Read the model definition and answer for the solid it produces. Units are mm, in the model's axes. A direction names the side the tool comes from. Coordinates: 2 decimals unless noted, no trailing zeros. Write each loop counter-clockwise with the first axis right and the second up, starting at its lowest first coordinate (ties: lowest second). Pieces come first, ordered by that corner, then holes. Notation, with made-up numbers: (-30.75, -24) -> (15.25, -24) arc R23 cw to (15.25, 11) -> close; hole circle Ø4 at (17, -32.5). An arc over 180 degrees is marked (long way). One line per item, written item: value. Start each with the question number.
1. Find section A-A, the plane x = 31.5. Write down the section's boundary in (y, z).
2. For a pull along X with two mould halves and no side action, classify faces 1 (the flat face through (2, -62, 70)), 2 (the flat face through (0, -63, 35)), 3 (the flat face through (5, -120, 60.75)) as pulls with the +X half, pulls with the -X half, needs draft (parallel to the pull), parting line crosses it, or undercut.
3. Consider line 1 along Y through (x, z) = (4.75, 64.5); line 2 along X through (y, z) = (-48.5, 35); line 3 along Y through (x, z) = (30.5, 54). Determine where each line is inside the solid, lowest interval first.
4. For faces 4 (the cylindrical face through (1.5, -70.4, 31.3)), 5 (the cylindrical face through (13.65, -1.52, 34.71)), 6 (the flat face through (6, -119, 66.75)), determine the directions among +Z, -Z, +X, -X, +Y, -Y from which every point of the face is accessible in a straight line to the end or side of a thin tool.
5. Find section C-C, the plane y = -98. Write down the section's boundary in (x, z).
6. Find section B-B, the plane z = 56. Write down the section's boundary in (x, y).
7. Given P1, Ø0.6, axis at x = 9.5, y = -9, coming from the +Z side; P2, Ø1.6, axis at x = 90, y = -81, coming from the +Z side, each flat-ended and moving along its own axis, determine where each tip first touches the part or whether it passes through.
8. Find section D-D, the plane x = 75.5. Write down the section's boundary in (y, z).
Autodesk Inventor part; units mm, degrees
ref_plane "Plano de trabajo2" through (0, 0, 60.25) normal (0, 0, 1) x (1, 0, 0)
ref_plane "YZ Plane" through (0, 0, 0) normal (1, 0, 0) x (0, 1, 0)
ref_plane "XZ Plane" through (0, 0, 0) normal (0, 1, 0) x (-1, 0, 0)
sketch "Boceto3" plane through (0, 0, 0) normal (0, 0, 1) x (1, 0, 0)
  line L0 (0, 0) -> (100, 0)
  line L1 (100, 0) -> (100, -125)
  line L2 (100, -125) -> (0, -125)
  line L3 (0, -125) -> (0, 0)
  dimension "d8" = 100
  dimension "d9" = 125
extrude "Extrusión2" add sketch "Boceto3" along normal blind 70
sketch "Boceto4" plane through (0, 0, 70) normal (0, 0, 1) x (1, 0, 0)
  line L0 (0, 0) -> (50, 0)
  line L1 (100, 0) -> (0, 0)
  line L2 (0, 0) -> (0, -125)
  line L3 (0, 0) -> (0, -45)
  line L4 (6.25, -5.5) -> (93.75, -5.5)
  line L5 (93.75, -5.5) -> (93.75, -84.5)
  line L6 (93.75, -84.5) -> (6.25, -84.5)
  line L7 (6.25, -84.5) -> (6.25, -5.5)
  line L8 (6.25, -5.5) -> (93.75, -84.5) construction
  line L9 (93.75, -5.5) -> (6.25, -84.5) construction
  line L10 (6.25, -5.5) -> (9.75, -5.5)
  line L11 (6.25, -5.5) -> (6.25, -9)
  circle A0 centre (9.75, -9) radius 1
  line L12 (93.75, -5.5) -> (90.25, -5.5)
  line L13 (93.75, -5.5) -> (93.75, -9)
  circle A1 centre (90.25, -9) radius 1
  line L14 (93.75, -84.5) -> (90.25, -84.5)
  line L15 (93.75, -84.5) -> (93.75, -81)
  circle A2 centre (90.25, -81) radius 1
  line L16 (6.25, -84.5) -> (9.75, -84.5)
  line L17 (6.25, -84.5) -> (6.25, -81)
  circle A3 centre (9.75, -81) radius 1
  point P0 (50, -45)
  dimension "d12" = 45
  dimension "d13" = 87.5
  dimension "d14" = 79
  dimension "d22" = 3.5
  dimension "d23" = 3.5
  dimension "d24" = 2
  dimension "d25" = 3.5
  dimension "d26" = 3.5
  dimension "d27" = 2
  dimension "d28" = 3.5
  dimension "d29" = 3.5
  dimension "d30" = 2
  dimension "d31" = 3.5
  dimension "d32" = 3.5
  dimension "d33" = 2
sketch "Boceto5" plane through (0, 0, 70) normal (0, 0, 1) x (1, 0, 0)
  line L0 (100, 0) -> (0, 0)
  line L1 (0, 0) -> (0, -62.5)
  line L2 (0, 0) -> (0, -125)
  line L3 (0, 0) -> (3, 0)
  line L4 (0, 0) -> (0, -3)
  line L5 (100, -125) -> (100, 0)
  line L6 (100, -125) -> (100, -122)
  line L7 (0, -125) -> (100, -125)
  line L8 (100, -125) -> (97, -125)
  line L9 (97, -122) -> (3, -122)
  line L10 (3, -122) -> (3, -3)
  line L11 (3, -3) -> (97, -3)
  line L12 (97, -3) -> (97, -122)
  dimension "d15" = 62.5
  dimension "d16" = 3
  dimension "d17" = 3
  dimension "d18" = 3
  dimension "d19" = 3
extrude "Extrusión3" cut sketch "Boceto5" against normal blind 60 contours L9 L10 L11 L12
extrude "Extrusión4" cut sketch "Boceto4" against normal blind 65 contours A0 | A1 | A2 | A3
sketch "Boceto7" plane through (0, 0, 70) normal (0, 0, 1) x (1, 0, 0)
  point P0 (0, 0)
sketch "Boceto8" plane through (0, 0, 70) normal (0, 0, 1) x (1, 0, 0)
  point P0 (0, 0)
ref_plane "Plano de trabajo1" through (0, 0, 60.75) normal (0, 0, 1) x (1, 0, 0)
sketch "Boceto9" plane through (0, 0, 60.75) normal (0, 0, 1) x (1, 0, 0)
  line L0 (3, -3) -> (6.5, -3)
  line L1 (6.5, -3) -> (6.5, -6.5)
  line L2 (6.5, -6.5) -> (3, -6.5)
  line L3 (3, -6.5) -> (3, -3)
  line L4 (97.0016, -3) -> (93.5016, -3)
  line L5 (93.5016, -3) -> (93.5016, -6.5)
  line L6 (93.5016, -6.5) -> (97.0016, -6.5)
  line L7 (97.0016, -6.5) -> (97.0016, -3)
  line L8 (3, -122) -> (3, -3)
  line L9 (3, -122) -> (6.5, -122)
  line L10 (6.5, -122) -> (6.5, -118.5)
  line L11 (6.5, -118.5) -> (3, -118.5)
  line L12 (3, -118.5) -> (3, -122)
  line L13 (97, -3) -> (97, -122)
  line L14 (97, -122) -> (93.5, -122)
  line L15 (93.5, -122) -> (93.5, -118.5)
  line L16 (93.5, -118.5) -> (97, -118.5)
  line L17 (97, -118.5) -> (97, -122)
  point P0 (0, 0)
  point P1 (97, -6.5)
  dimension "d61" = 3.5
  dimension "d62" = 3.5
  dimension "d63" = 3.5
  dimension "d64" = 3.5
  dimension "d65" = 3.5
  dimension "d66" = 3.5
  dimension "d70" = 3.5
  dimension "d71" = 3.5
ref_plane "Plano de trabajo2" through (0, 0, 60.25) normal (0, 0, 1) x (1, 0, 0)
sketch "Boceto10" plane through (3, -122, 70) normal (0, 1, 0) x (1, 0, 0)
  point P0 (-3, 70)
sketch "Boceto11" plane through (0, 0, 10) normal (0, 0, 1) x (1, 0, 0)
  line L0 (-58.2651, -184.2292) -> (-60.7624, -188.5609)
  point P0 (0, 0)
  dimension "d68" = 5
sketch "Boceto12" plane through (0, 0, 60.75) normal (0, 0, 1) x (1, 0, 0)
  point P0 (0, 0)
extrude "Extrusión6" add sketch "Boceto9" along normal blind 6
sketch "Boceto13" plane through (0, 0, 66.75) normal (0, 0, 1) x (1, 0, 0)
  point P0 (0, 0)
sketch "Boceto14" plane through (0, 0, 66.75) normal (0, 0, 1) x (1, 0, 0)
  line L0 (6.5, -122) -> (6.5, -118.5)
  line L1 (6.5, -118.5) -> (4.75, -118.5)
  line L2 (6.5, -118.5) -> (3, -118.5)
  line L3 (6.5, -118.5) -> (6.5, -120.25)
  circle A0 centre (4.75, -120.25) radius 1
  line L4 (93.5, -118.5) -> (93.5, -122)
  line L5 (93.5, -118.5) -> (95.25, -118.5)
  line L6 (97, -118.5) -> (93.5, -118.5)
  line L7 (93.5, -118.5) -> (93.5, -120.25)
  circle A1 centre (95.25, -120.25) radius 1
  line L8 (3, -3) -> (97, -3)
  line L9 (97, -3) -> (95.25, -3)
  line L10 (97, -3) -> (97, -4.75)
  line L11 (97, -3) -> (97, -122)
  circle A2 centre (95.25, -4.75) radius 1
  line L12 (3, -122) -> (3, -3)
  line L13 (3, -3) -> (4.75, -3)
  line L14 (3, -3) -> (3, -4.75)
  circle A3 centre (4.75, -4.75) radius 1
  point P0 (0, 0)
  dimension "d74" = 1.75
  dimension "d75" = 1.75
  dimension "d76" = 2
  dimension "d77" = 1.75
  dimension "d78" = 1.75
  dimension "d79" = 2
  dimension "d80" = 1.75
  dimension "d81" = 1.75
  dimension "d82" = 2
  dimension "d83" = 1.75
  dimension "d84" = 1.75
  dimension "d85" = 2
extrude "Extrusión7" cut sketch "Boceto14" against normal blind 4
sketch "Boceto15" plane through (0, 0, 66.75) normal (0, 0, 1) x (1, 0, 0)
  point P0 (0, 0)
sketch "Boceto16" plane through (3, -122, 70) normal (1, 0, 0) x (0, 0, -1)
  line L0 (60, 0) -> (60, 119)
  line L1 (60, 50.4292) -> (40, 50.4292)
  line L2 (60, 50.4292) -> (80, 50.4292) construction
  circle A0 centre (40, 50.4292) radius 1.75
  line L3 (40, 50.4292) -> (40, 55.4292)
  circle A1 centre (40, 55.4292) radius 1.75
  point P0 (70, 122)
  dimension "d88" = 20
  dimension "d89" = 180
  dimension "d90" = 3.5
  dimension "d91" = 5
  dimension "d92" = 3.5
extrude "Extrusión8" cut sketch "Boceto16" against normal blind 10
sketch "Boceto17" plane through (3, -3, 70) normal (0, -1, 0) x (1, 0, 0)
  line L0 (0, -60) -> (94, -60)
  line L1 (23.6532, -59.4188) -> (73.6532, -59.4188) construction
  circle A0 centre (23.6532, -9.4188) radius 1.75
  circle A1 centre (28.6532, -9.4188) radius 1.75
  circle A2 centre (33.6532, -9.4188) radius 1.75
  circle A3 centre (38.6532, -9.4188) radius 1.75
  circle A4 centre (53.6532, -9.4188) radius 1.75
  point P0 (-3, -70)
  dimension "d97" = 3.5
  dimension "d99" = 3.5
  dimension "d101" = 3.5
  dimension "d103" = 3.5
  dimension "d109" = 3.5
extrude "Extrusión9" cut sketch "Boceto17" against normal blind 10
sketch "Boceto18" plane through (3, -3, 70) normal (0, -1, 0) x (1, 0, 0)
  line L0 (0, -60) -> (94, -60)
  line L1 (11.2664, -60) -> (31.2664, -60) construction
  circle A0 centre (11.2664, -40) radius 4.75
  point P0 (-3, -70)
  dimension "d114" = 9.5
extrude "Extrusión10" cut sketch "Boceto18" against normal blind 10
properties part number "base"
Answer block:
1. outline: (-125, 0) -> (0, 0) -> (0, 58.84) -> (-3, 58.84) -> (-3, 10) -> (-122, 10) -> (-122, 70) -> (-125, 70) -> close; (-3, 62.32) -> (0, 62.32) -> (0, 70) -> (-3, 70) -> close
2. face 1: needs draft
2. face 2: pulls with the -X half
2. face 3: undercut
3. line 1: y = -125 to -121.25, -119.25 to -118.5, -6.5 to -5.75, -3.75 to 0
3. line 2: x = 0 to 3, 97 to 100
3. line 3: y = -125 to -122, -3 to 0
4. face 4: -X
4. face 5: +Y
4. face 6: +Z
5. outline: (0, 0) -> (100, 0) -> (100, 70) -> (97, 70) -> (97, 10) -> (3, 10) -> (3, 70) -> (0, 70) -> close
6. outline: (0, -125) -> (100, -125) -> (100, 0) -> (0, 0) -> close; hole (3, -122) -> (97, -122) -> (97, -3) -> (3, -3) -> close
7. P1: stops at z = 5
7. P2: stops at z = 10
8. outline: (-125, 0) -> (0, 0) -> (0, 70) -> (-3, 70) -> (-3, 10) -> (-122, 10) -> (-122, 70) -> (-125, 70) -> close
